Part model, mm, in its own coordinate system. A direction names the side the tool comes from. Coordinates: 2 decimals unless noted, no trailing zeros. Order: outer loops, then holes, each group sorted by start corner. A loop starts at its lowest first (then second) coordinate and runs counter-clockwise, first axis right, second up.
from build123d import *

# Parameters (mm, degrees)
SKETCH1_R           = 1.5
BOSS_EXTRUDE1_DEPTH = 3
SKETCH2_W           = 40.53
SKETCH2_H           = 6
CUT_EXTRUDE1_DEPTH  = 1


with BuildPart() as part:
    # Sketch1 → Boss-Extrude1 (new body)
    with BuildSketch(Plane(origin=(0, 0, 0), x_dir=(0, 0, -1), z_dir=(1, 0, 0))):
        with BuildLine():
            Line((0, -3), (40.53, -3))
            ThreePointArc((40.53, -3), (43.53, 0), (40.53, 3))
            Line((40.53, 3), (0, 3))
            ThreePointArc((0, 3), (-3, 0), (0, -3))
        make_face()
        Circle(SKETCH1_R, mode=Mode.SUBTRACT)
        with Locations((40.53, 0)):
            Circle(SKETCH1_R, mode=Mode.SUBTRACT)
    extrude(amount=BOSS_EXTRUDE1_DEPTH)

    # Sketch2 → Cut-Extrude1 (cut)
    with BuildSketch(Plane.ZY):
        with Locations((-23.265, 0)):
            Rectangle(SKETCH2_W, SKETCH2_H)
    extrude(amount=-CUT_EXTRUDE1_DEPTH, mode=Mode.SUBTRACT)


solid = part.part
Q1. Pin check, flat tips, straight feed: pin 1 Ø2 at (y, z) = (0.5, -8.5) entering from -X; pin 2 Ø1.8 at (y, z) = (0, 0) entering from +X. Stop position of each tip, or through.
Results list:
pin 1: stops at x = 1
pin 2: passes through
Q2. Mould opens along Z. For faces 1 (the face through (2, 3, -21)), 2 (the face through (1.99, 0.45, -41.96)), 3 (the face through (1.99, -0.07, -43.53)) say: pulls with the +Z half, pulls with the -Z half, needs draft (parallel to the pull), parting line crosses it, or undercut.
Results list:
face 1: needs draft
face 2: undercut
face 3: pulls with the -Z half
Q3. Cut at C-C on y = 2.4. Write the cut outline in (x, z), and give its area (3 significant figures).
Results list:
outline: (0, -3) - (1, -3) - (1, -42.33) - (3, -42.33) - (3, 1.8) - (0, 1.8) - close
area: 93.1 mm2
Q4. Which spindle directions (+Z, -Z, +X, -X, +Y, -Y) get a long thin tool onto all of the face, cutting with end or side? Do faces 4 (the face through (1, 0, -24)), 5 (the face through (3, 0, -20)). Say none if no direction does.
Results list:
face 4: -Z, -X, +Y, -Y
face 5: +Z, -Z, +X, +Y, -Y
Q5. Cut at B-B on x = 1.85. Write the cut outline in (y, z).
Results list:
outline: (-3, -40.53) arc R3 ccw to (3, -40.53) - (3, 0) arc R3 ccw to (-3, 0) - close; hole circle Ø3 at (0, -40.53); hole circle Ø3 at (0, 0)
Q6. Cut at A-A on y = 0. Write the cut outline in (x, z).
Results list:
outline: (0, -3) - (1, -3) - (1, -39.03) - (3, -39.03) - (3, -1.5) - (0, -1.5) - close; (0, 1.5) - (3, 1.5) - (3, 3) - (0, 3) - close; (1, -43.53) - (3, -43.53) - (3, -42.03) - (1, -42.03) - close
Q7. Wall check: line 1 along Z through (x, y) = (2.3, -0.05); line 2 along Y through (x, z) = (1, 0); line 3 along X through (y, z) = (-1.5, -37). Give the ranges that are in metal, low to high.
Results list:
line 1: z = -43.53 to -42.03, -39.03 to -1.5, 1.5 to 3
line 2: y = -3 to -1.5, 1.5 to 3
line 3: x = 1 to 3
Q8. Cut at D-D on z = -15. Write the cut outline in (x, y).
Results list:
outline: (1, -3) - (3, -3) - (3, 3) - (1, 3) - close
